Input: dimensioned drawing with shaded views. Units: mm. Origin: part minimum x, y, z. A direction names the side the tool comes from. Round coordinates to 2 decimals unless told otherwise and drop trailing zeros. Loops run counter-clockwise (first coordinate to the right, second up) from the corner with the lowest first, then second, coordinate; pieces in that order, holes last. Notation, with made-up numbers: M 79.5,-18 L 91.5,-18 A14 ccw 91.5,-14 Z; hole C -4,54.5 d9. An arc over 180 degrees is marked long. Return JSON: item names as keys, results as strings.
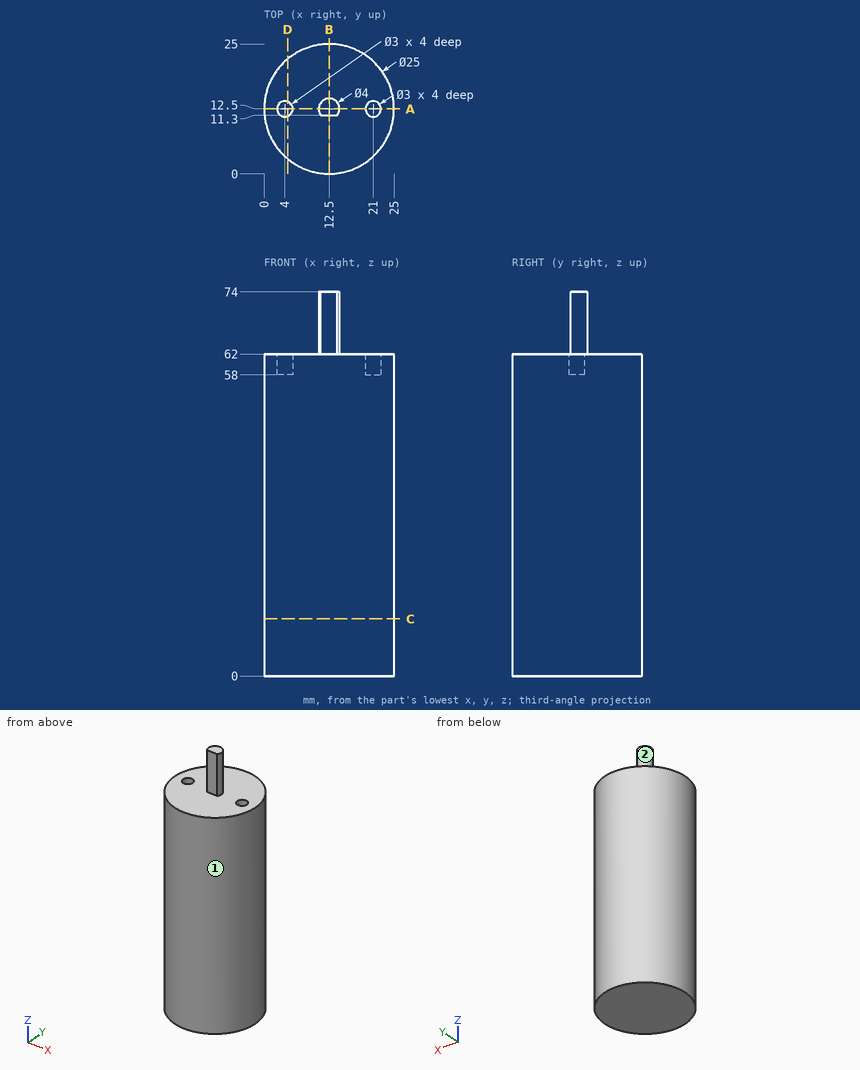
Q1. Pin query (flat end, axial travel): pin 1 (1.5 mm diameter, centred on x = 10.5, y = 21, fed in from +Z); pin 2 (5 mm diameter, centred on y = 6, z = 63.5, fed in from -X); pin 3 (12 mm diameter, centred on y = 22, z = 46.5, fed in from -X). Return the tip coordinate at first contact, or that it passes through.
Determined:
{"pin 1": "stops at z = 62", "pin 2": "stops at x = 0.84", "pin 3": "stops at x = 0.5"}
Q2. Section query D-D (x = 4.5). Output: boundary loops of the cut face in (y, z), plus the area to 3 significant figures.
Determined:
{"outline": "M 2.9,0 L 22.1,0 L 22.1,62 L 13.91,62 L 13.91,58 L 11.09,58 L 11.09,62 L 2.9,62 Z", "area": "1,180 mm^2"}
Q3. Section query C-C (z = 11). Output: boundary loops of the cut face in (x, y).
Determined:
{"outline": "C 12.5,12.5 d25"}
Q4. Reachability of the marked faces 1 and 2 from +Z, -Z, +X, -X, +Y, -Y: full face, straight path, thin tool, end or side. Return the list, or none.
Determined:
{"face 1": "+Z, -Z", "face 2": "+Z"}
Q5. Section query B-B (x = 12.5). Output: boundary loops of the cut face in (y, z), plus the area to 3 significant figures.
Determined:
{"outline": "M 0,0 L 25,0 L 25,62 L 14.5,62 L 14.5,74 L 11.3,74 L 11.3,62 L 0,62 Z", "area": "1,590 mm^2"}
Q6. Section query A-A (y = 12.5). Output: boundary loops of the cut face in (x, z).
Determined:
{"outline": "M 0,0 L 25,0 L 25,62 L 22.5,62 L 22.5,58 L 19.5,58 L 19.5,62 L 14.5,62 L 14.5,74 L 10.5,74 L 10.5,62 L 5.5,62 L 5.5,58 L 2.5,58 L 2.5,62 L 0,62 Z"}
Q7. Material intervals for L1, parallel to Z at x = 21.25, y = 19.5; L2, parallel to Y at x = 21, z = 58.9; L3, parallel to Y at x = 12, z = 61.5, sorted ascending.
Determined:
{"L1": "z = 0 to 62", "L2": "y = 3.33 to 11, 14 to 21.67", "L3": "y = 0.01 to 24.99"}
